For this review, take the finished solid that the model builds, in its own axes (mm). Round coordinates to 2 decimals unless told otherwise and drop trailing zeros. Order: outer loops, then holes, each group sorted by start corner. A loop starts at its lowest first (then second) coordinate and runs counter-clockwise, first axis right, second up. Notation, with made-up numbers: (6.5, 64.25) -> (38.5, 64.25) arc R25 ccw to (38.5, 85.25) -> close; hole circle Ø4 at (53, 49.25). An arc over 180 degrees is marked (long way). Use a Markdown table: item, result. Add a question column.
1) Clearance check with a flat-ended pin moving along its axis: P1, Ø3, axis at y = 5, z = 0.5, coming from the -X side. State where the tip first meets the part, or that it passes through.
2) Consider section A-A (y = 0). State the section outline as (x, z) points, plus the area to 4 significant figures.
3) Wall thickness on line 1 along Y through (x, z) = (0, 2); line 2 along Y through (x, z) = (-25.5, 2.45); line 3 along X through (y, z) = (-27.5, -0.3): over which ranges is each line inside the solid? List them lowest first. Write a range as [from, to].
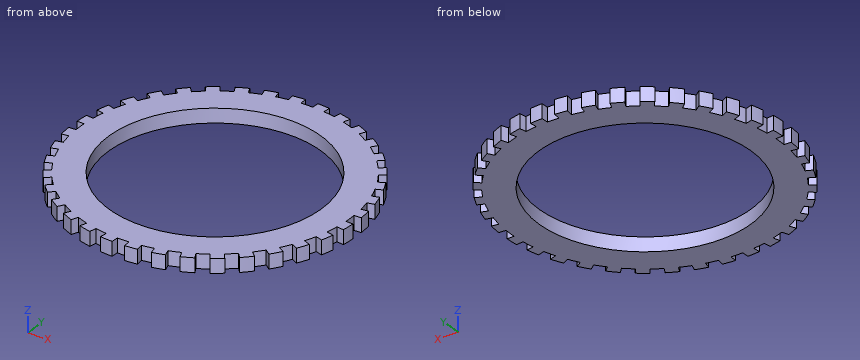
```python
from build123d import *

# Parameters (mm, degrees)
SKETCH1_R           = 20
SKETCH1_R_2         = 15
BOSS_EXTRUDE1_DEPTH = 2
CUT_EXTRUDE1_START  = -2
CUT_EXTRUDE1_DEPTH  = 2
CIRPATTERN1_COUNT   = 36
SCALE1_SCALE        = 1.9329
SCALE2_SCALE        = 1.5


with BuildPart() as part:
    # Sketch1 → Boss-Extrude1 (new body)
    with BuildSketch(Plane.XY):
        Circle(SKETCH1_R)
        Circle(SKETCH1_R_2, mode=Mode.SUBTRACT)
    extrude(amount=BOSS_EXTRUDE1_DEPTH)

    # Sketch2 → Cut-Extrude1 (cut)
    with BuildSketch(Plane.XY.offset(2).offset(CUT_EXTRUDE1_START)):
        with BuildLine():
            Line((-18.47787485, -4.423589156), (-19.450394579, -4.656409638))
            ThreePointArc((-19.450394579, -4.656409638), (-19.634991849, -3.803563472), (-19.782212796, -2.943477007))
            Line((-19.782212796, -2.943477007), (-18.793102156, -2.796303156))
            ThreePointArc((-18.793102156, -2.796303156), (-18.653242257, -3.613385298), (-18.47787485, -4.423589156))
        make_face()
    cut_extrude1 = extrude(amount=CUT_EXTRUDE1_DEPTH, mode=Mode.SUBTRACT)

    # CirPattern1: Cut-Extrude1 ×36 about axis
    cirpattern1_axis = Axis((0, 0, 0), (0, 0, 1))
    for i in range(1, CIRPATTERN1_COUNT):
        add(cut_extrude1.rotate(cirpattern1_axis, i * 360 / CIRPATTERN1_COUNT), mode=Mode.SUBTRACT)


with BuildPart() as part_1:
    # Scale1: scaled about (0, 0, 1)
    add(part.part.scale(SCALE1_SCALE).moved(Location((0, 0, -0.9329))))


with BuildPart() as part_2:
    # Scale2: scaled about (0, 0, 1)
    add(part_1.part.scale(SCALE2_SCALE).moved(Location((0, 0, -0.5))))


solid = part_2.part
```
Results list:
| question | item | result |
|---|---|---|
| 1 | P1 | x = -57.88 |
| 2 | outline | (-55.09, -1.9) -> (-43.49, -1.9) -> (-43.49, 3.9) -> (-55.09, 3.9) -> close; (43.49, -1.9) -> (55.09, -1.9) -> (55.09, 3.9) -> (43.49, 3.9) -> close |
| 2 | area | 134.5 mm2 |
| 3 | line 1 | [-55.09, -43.49], [43.49, 55.09] |
| 3 | line 2 | [-52.08, -51.06], [-48.83, -35.23], [35.23, 52.08] |
| 3 | line 3 | [-51.05, -50.73], [-47.73, -33.69], [33.69, 47.73] |
